Design review of the part built by this model. Coordinates are the model's own, in mm. A direction names the side the tool comes from. Coordinates: 2 decimals unless noted, no trailing zeros. Loops run counter-clockwise (first coordinate to the right, second up) from the corner with the lowest first, then second, coordinate; pieces in that order, holes last. Notation, with made-up numbers: (55, 25.25) -> (66, 25.25) arc R10 ccw to (66, 38.25) -> close; hole circle Ø3 at (81.25, 29). An arc over 180 degrees is marked (long way). One line per item, written item: value. Start each with the question number.
1. Add section D-D on x = -28. Write out the cut boundary in (y, z), plus the area to 3 significant figures.
2. Add section C-C on x = 15. Write out the cut boundary in (y, z) (3 decimals), plus the area to 3 significant figures.
3. Add section A-A on y = 10. Write out the cut boundary in (x, z) (3 decimals), plus the area to 3 significant figures.
4. Insertion check: pin 1 (5 mm diameter, centred on y = 6, z = -20, fed in from +X); pin 2 (5 mm diameter, centred on y = 6, z = -10.5, fed in from -X); pin 3 (2.5 mm diameter, centred on x = -15.5, z = 13.5, fed in from +Y). Each pin has a flat end and moves straight along its axis. Give the tip position at first contact, or say it passes through.
5. Machinability: for faces 4 (the flat face through (-15, 15, -10)), 5 (the cylindrical face through (-7.74, 8.92, -16.61)), which of the approach directions +Z, -Z, +X, -X, +Y, -Y give a long, thin tool a straight path to every point of the face, cutting with its end or side? Answer none if there is none.
6. Draft analysis for pull direction X (two halves, no side actions). For faces 1 (the flat face through (-15, 3, 15)), 2 (the flat face through (40, 1, 1)), 3 (the flat face through (-1, 0, -1)), state which applies: pulls with the +X half, pulls with the -X half, needs draft (parallel to the pull), parting line crosses it, or undercut.
7. For probe 1 along X at (y, z) = (7.5, -15) (3 decimals); probe 2 along Y at (x, z) = (-13.5, 11); probe 3 along X at (y, z) = (8.5, 20.5), list the stretches that pass through material, from the lowest coordinate up.
8. Add section B-B on z = 15. Write out the cut boundary in (x, y) (3 decimals), plus the area to 3 significant figures.
```python
from build123d import *

# Parameters (mm, degrees)
SKETCH1_W                 = 80
SKETCH1_H                 = 80
BOSS_EXTRUDE1_DEPTH       = 3
SKETCH2_R                 = 7.435
SKETCH2_R_2               = 4.435
BOSS_EXTRUDE2_DEPTH       = 12
MIRROR2_COPY_1_SKETCH_R   = 7.435
MIRROR2_COPY_1_SKETCH_R_2 = 4.435
MIRROR2_COPY_1_DEPTH      = 12


with BuildPart() as part:
    # Sketch1 → Boss-Extrude1 (new body)
    with BuildSketch(Plane(origin=(0, 0, 0), x_dir=(1, 0, 0), z_dir=(0, 1, 0))):
        Rectangle(SKETCH1_W, SKETCH1_H)
    extrude(amount=BOSS_EXTRUDE1_DEPTH)

    # Sketch2 → Boss-Extrude2 (add)
    with BuildSketch(Plane(origin=(0, 3, 0), x_dir=(1, 0, 0), z_dir=(0, 1, 0))):
        with Locations(Location((-15, -15, 0), (0, 0, 90))):  # turned: the seam where the file's is
            Circle(SKETCH2_R)
        with Locations(Location((-15, -15, 0), (0, 0, 270))):  # turned: the seam where the file's is
            Circle(SKETCH2_R_2, mode=Mode.SUBTRACT)
    boss_extrude2 = extrude(amount=BOSS_EXTRUDE2_DEPTH)

    # Mirror1: Boss-Extrude2 across plane
    add(boss_extrude2.mirror(Plane.XY))

    # Mirror2: Boss-Extrude2 across plane
    add(boss_extrude2.mirror(Plane(origin=(0, 0, 0), x_dir=(0, 0, 1), z_dir=(1, 0, 0))))

    # Mirror2 copy 1 sketch → Mirror2 copy 1 (add)
    with BuildSketch(Plane(origin=(0, 3, 0), x_dir=(-1, 0, 0), z_dir=(0, 1, 0))):
        with Locations(Location((-15, -15, 0), (0, 0, 90))):  # turned: the seam where the file's is
            Circle(MIRROR2_COPY_1_SKETCH_R)
        with Locations(Location((-15, -15, 0), (0, 0, 270))):  # turned: the seam where the file's is
            Circle(MIRROR2_COPY_1_SKETCH_R_2, mode=Mode.SUBTRACT)
    extrude(amount=MIRROR2_COPY_1_DEPTH)


solid = part.part
```
Worked answers:
1. outline: (0, -40) -> (3, -40) -> (3, 40) -> (0, 40) -> close
1. area: 240 mm²
2. outline: (0, -40) -> (3, -40) -> (3, -22.435) -> (15, -22.435) -> (15, -19.435) -> (3, -19.435) -> (3, -10.565) -> (15, -10.565) -> (15, -7.565) -> (3, -7.565) -> (3, 7.565) -> (15, 7.565) -> (15, 10.565) -> (3, 10.565) -> (3, 19.435) -> (15, 19.435) -> (15, 22.435) -> (3, 22.435) -> (3, 40) -> (0, 40) -> close
2. area: 384 mm²
3. outline: circle Ø14.87 at (-15, -15); circle Ø14.87 at (-15, 15); circle Ø14.87 at (15, -15); circle Ø14.87 at (15, 15); hole circle Ø8.87 at (-15, -15); hole circle Ø8.87 at (-15, 15); hole circle Ø8.87 at (15, -15); hole circle Ø8.87 at (15, 15)
3. area: 447 mm²
4. pin 1: stops at x = 22
4. pin 2: stops at x = -22.16
4. pin 3: stops at y = 3
5. face 4: +Z, -Z, +X, -X, +Y
5. face 5: +Y
6. face 1: undercut
6. face 2: pulls with the +X half
6. face 3: needs draft
7. probe 1: x = -22.435 to -19.435, -10.565 to -7.565, 7.565 to 10.565, 19.435 to 22.435
7. probe 2: y = 0 to 3
7. probe 3: x = -20 to -10, 10 to 20
8. outline: (-40, 0) -> (40, 0) -> (40, 3) -> (22.435, 3) -> (22.435, 15) -> (19.435, 15) -> (19.435, 3) -> (10.565, 3) -> (10.565, 15) -> (7.565, 15) -> (7.565, 3) -> (-7.565, 3) -> (-7.565, 15) -> (-10.565, 15) -> (-10.565, 3) -> (-19.435, 3) -> (-19.435, 15) -> (-22.435, 15) -> (-22.435, 3) -> (-40, 3) -> close
8. area: 384 mm²
